from build123d import *

# Parameters (mm, degrees)
SKETCH1_R           = 2.413
BOSS_EXTRUDE1_DEPTH = 3.175
BOSS_EXTRUDE2_DEPTH = 5.08
SKETCH4_W           = 4
SKETCH4_H           = 24.78484928
CUT_EXTRUDE2_DEPTH  = 5.08
FILLET1_R           = 0.635
SKETCH5_R           = 4.1275
CUT_EXTRUDE3_DEPTH  = 5.08


with BuildPart() as part:
    # Sketch1 → Boss-Extrude1 (new body)
    with BuildSketch(Plane.XY):
        with BuildLine():
            Line((0, 20.591373255), (-38.1, 20.591373255))
            Line((-38.1, 20.591373255), (-38.1, 10.208864232))
            ThreePointArc((-38.1, 10.208864232), (-19.722011237, 2.596452037), (0, 0))
            Line((0, 0), (0, 20.591373255))
        make_face()
        with Locations((-10.16, 9.398)):
            Circle(SKETCH1_R, mode=Mode.SUBTRACT)
        with Locations((-22.86, 9.398)):
            Circle(SKETCH1_R, mode=Mode.SUBTRACT)
    extrude(amount=BOSS_EXTRUDE1_DEPTH)

    # Sketch2 → Boss-Extrude2 (add)
    with BuildSketch(Plane.XY.offset(3.175)):
        Polygon((-38.1, 15.846028276), (-17.78, 14.075883223), (-17.78, 11.782028276), (-38.1, 11.782028276), align=None)
        Polygon((-17.78, 17.286663737), (-34.332210433, 18.728583688), (-35.56, 19.956373255), (-35.56, 20.591373255), (-17.78, 20.591373255), align=None)
    extrude(amount=BOSS_EXTRUDE2_DEPTH)

    # Sketch4 → Cut-Extrude2 (cut)
    with BuildSketch(Plane.XY.offset(3.175)):
        with Locations((-2, 12.39242464)):
            Rectangle(SKETCH4_W, SKETCH4_H)
    extrude(amount=-CUT_EXTRUDE2_DEPTH, mode=Mode.SUBTRACT)

    # Fillet1
    fillet1_edges = [part.edges().sort_by_distance(p)[0] for p in [
        (-4, 0.105059301, 1.5875),
        (-38.1, 10.208864232, 1.5875),
    ]]
    fillet(fillet1_edges, radius=FILLET1_R)

    # Sketch5 → Cut-Extrude3 (cut)
    with BuildSketch(Plane.XY.offset(8.255)):
        with Locations((-22.86, 9.398)):
            Circle(SKETCH5_R)
    extrude(amount=-CUT_EXTRUDE3_DEPTH, mode=Mode.SUBTRACT)


solid = part.part
Work out the finished part from the listing and answer in its coordinate system (mm). A direction names the side the tool comes from. Round coordinates to 2 decimals unless told otherwise and drop trailing zeros. Order: outer loops, then holes, each group sorted by start corner. A loop starts at its lowest first (then second) coordinate and runs counter-clockwise, first axis right, second up. Notation, with made-up numbers: M -4.5,6 L 45.5,6 A14 cw 45.5,23 Z; hole C 13.25,41 d11. An arc over 180 degrees is marked long. One line per item, written item: value.
Q1. Determine the mould class of faces 6 (the face through (-25, 20.591, 3)), 7 (the face through (-34.938, 19.334, 5.679)), 8 (the face through (-19, 11.782, 6)) for opening direction Y: released by +Y, released by -Y, zero draft, split by the parting line, or undercut.
Derived:
face 6: released by +Y
face 7: undercut
face 8: released by -Y
Q2. Find section D-D on z = 1.5. Write down the section's boundary in (x, y) (1 decimal).
Derived:
outline: M -38.1,10.6 A0.6 ccw -37.8,10 A76.2 ccw -4.7,0.1 A0.6 ccw -4,0.8 L -4,20.6 L -38.1,20.6 Z; hole C -22.9,9.4 d4.8; hole C -10.2,9.4 d4.8
Q3. Find section B-B on x = -9. Write down the section's boundary in (y, z) (3 decimals), then the cut area to 3 significant figures.
Derived:
outline: M 0.533,0 L 7.282,0 L 7.282,3.175 L 0.533,3.175 Z; M 11.514,0 L 20.591,0 L 20.591,3.175 L 11.514,3.175 Z
area: 50.2 mm²
Q4. Flat-ended cylindrical pins translate along their axes: pin 1 (4 mm diameter, centred on x = -17, z = 7, fed in from -Y); pin 2 (1 mm diameter, centred on y = 19, z = 7, fed in from +X); pin 3 (0.7 mm diameter, centred on y = 20.5, z = 5.5, fed in from -X). Find the tip coordinate at first contact, or state that the pin passes through.
Derived:
pin 1: y = 11.78
pin 2: x = -17.78
pin 3: x = -35.56
Q5. Straight lines are drawn through the part: line 1 (X direction, y = 8.5, z = 3); line 2 (Z direction, x = -16.5, y = 14) (3 decimals); line 3 (X direction, y = 7.5, z = 2.5). For each, find the intervals that lie inside material, in ascending order.
Derived:
line 1: -34.97 to -25.1, -20.62 to -12.4, -7.92 to -4
line 2: 0 to 3.175
line 3: -32.97 to -24.35, -21.37 to -11.65, -8.67 to -4
Q6. Find section C-C on y = 7.75. Write down the section's boundary in (x, z) (3 decimals).
Derived:
outline: M -33.482,0 L -24.623,0 L -24.623,3.175 L -33.482,3.175 Z; M -21.097,0 L -11.923,0 L -11.923,3.175 L -21.097,3.175 Z; M -8.397,0 L -4,0 L -4,3.175 L -8.397,3.175 Z
Q7. Find section A-A on z = 7.75. Write down the section's boundary in (x, y) (1 decimal).
Derived:
outline: M -38.1,11.8 L -26.2,11.8 A4.1 cw -19.5,11.8 L -17.8,11.8 L -17.8,14.1 L -38.1,15.8 Z; M -35.6,20 L -34.3,18.7 L -17.8,17.3 L -17.8,20.6 L -35.6,20.6 Z
Q8. For faces 1 (the face through (-28.082, 14.973, 5.679)), 2 (the face through (-17.78, 19, 6)), 3 (the face through (-32, 11.782, 6)), 4 (the face through (-25.94, 17.998, 5.679)), 5 (the face through (-22.805, 13.525, 5.751)), determine the directions among +Z, -Z, +X, -X, +Y, -Y from which every point of the face is accessible in a straight line to the end or side of a thin tool.
Derived:
face 1: +Z, +X
face 2: +Z, +X, +Y, -Y
face 3: +Z, +X, -X, -Y
face 4: +Z, -X
face 5: +Z, -Y
